```python
from build123d import *

# Parameters (mm, degrees)
SKETCH_1_W        = 30
SKETCH_1_H        = 30
EXTRUDE_268_DEPTH = 22
SKETCH_2_R        = 5.875
EXTRUDE_2_DEPTH   = 14.4
SKETCH_4_R        = 2.4
EXTRUDE_3_DEPTH   = 15.6


with BuildPart() as part:
    # Эскиз1 → Extrude 268 (new body)
    with BuildSketch(Plane(origin=(0, 0, 0), x_dir=(1, 0, 0), z_dir=(0, 1, 0))):
        with Locations((-1.294416244, -1.751269036)):
            Rectangle(SKETCH_1_W, SKETCH_1_H)
    extrude(amount=EXTRUDE_268_DEPTH)

    # Эскиз2 → Бобышка-Вытянуть2 (add)
    with BuildSketch(Plane(origin=(0, 22, 0), x_dir=(1, 0, 0), z_dir=(0, 1, 0))):
        with Locations(Location((0, 0, 0), (0, 0, 270))):
            Circle(SKETCH_2_R)
    extrude(amount=EXTRUDE_2_DEPTH)

    # Эскиз4 → Бобышка-Вытянуть3 (add)
    with BuildSketch(Plane(origin=(0, 36.4, 0), x_dir=(1, 0, 0), z_dir=(0, 1, 0))):
        with Locations(Location((0, 0, 0), (0, 0, 270))):
            Circle(SKETCH_4_R)
    extrude(amount=EXTRUDE_3_DEPTH)


solid = part.part
```
CAD build for the part. Positions are in the model's coordinates, mm. A direction names the side the tool comes from. Round coordinates to 2 decimals unless told otherwise and drop trailing zeros. Write each loop counter-clockwise with the first axis right and the second up, starting at its lowest first coordinate (ties: lowest second). Pieces come first, ordered by that corner, then holes. Notation, with made-up numbers: (-37, -24) - (4, -24) arc R20 ccw to (4, -14) - close; hole circle Ø9 at (-21, -37.5). An arc over 180 degrees is marked (long way). Return JSON: item names as keys, results as strings. Group by question number.
Item 1: Flat gauge pins, fed straight in: pin 1 Ø1.5 at (y, z) = (34, 0.5) entering from -X (3 decimals); pin 2 Ø10 at (x, y) = (-5.5, 35.5) entering from -Z; pin 3 Ø2 at (y, z) = (31, 5.5) entering from -X. Where does each tip first touch, or does it go through?
Item 2: Band-saw the part on B-B on z = 0. List the corners of the cut face in (x, y) (3 decimals), plus the area to 3 significant figures.
Item 3: 3-axis set-ups, long thin cutter, end or side, ignore diameter. For faces 1 (the face through (2.024, 44.091, 1.29)), 2 (the face through (13.706, 11, 2)): which of +Z, -Z, +X, -X, +Y, -Y reach the whole face in a straight line?
Item 4: Band-saw the part on D-D on x = 3.75. List the corners of the cut face in (y, z).
Item 5: Band-saw the part on A-A on x = 0. List the corners of the cut face in (y, z) (3 decimals), plus the area to 3 significant figures.
Item 6: Band-saw the part on C-C on y = 23.5. List the corners of the cut face in (x, z) (3 decimals).
Item 7: Probe probe 1 along Y at (x, z) = (4.75, 7.25); probe 2 along Z at (x, y) = (-0.75, 26); probe 3 along Z at (x, y) = (2.25, 26.5). List the from-to ranges inside material, lowest first.
Resolved:
{
 "1": {"pin 1": "stops at x = -5.875", "pin 2": "stops at z = -5.85", "pin 3": "stops at x = -3.78"},
 "2": {"outline": "(-16.294, 0) - (13.706, 0) - (13.706, 22) - (5.875, 22) - (5.875, 36.4) - (2.4, 36.4) - (2.4, 52) - (-2.4, 52) - (-2.4, 36.4) - (-5.875, 36.4) - (-5.875, 22) - (-16.294, 22) - close", "area": "904 mm²"},
 "3": {"face 1": "+Y", "face 2": "+Z, -Z, +X, +Y, -Y"},
 "4": {"outline": "(0, -13.25) - (22, -13.25) - (22, -4.52) - (36.4, -4.52) - (36.4, 4.52) - (22, 4.52) - (22, 16.75) - (0, 16.75) - close"},
 "5": {"outline": "(0, -13.249) - (22, -13.249) - (22, -5.875) - (36.4, -5.875) - (36.4, -2.4) - (52, -2.4) - (52, 2.4) - (36.4, 2.4) - (36.4, 5.875) - (22, 5.875) - (22, 16.751) - (0, 16.751) - close", "area": "904 mm²"},
 "6": {"outline": "circle Ø11.75 at (0, 0)"},
 "7": {"probe 1": "y = 0 to 22", "probe 2": "z = -5.83 to 5.83", "probe 3": "z = -5.43 to 5.43"}
}
